CAD build for the part. Positions are in the model's coordinates, mm. Face numbers are marked on the shaded views. A direction names the side the tool comes from. Give positions to 0.01 mm unless a question says otherwise; leave off trailing zeros. Write each loop counter-clockwise with the first axis right and the second up, starting at its lowest first coordinate (ties: lowest second). Pieces come first, ordered by that corner, then holes. Notation, with made-up numbers: (28.5, 42.5) -> (56.5, 42.5) arc R24 ccw to (56.5, 65.5) -> close; hole circle Ø6 at (16, -36). An arc over 180 degrees is marked (long way). Answer in a Markdown table with one row per item. Add a question column.
Autodesk Inventor part; units mm, degrees
ref_plane "YZ Plane" through (0, 0, 0) normal (1, 0, 0) x (0, 1, 0)
ref_plane "XZ Plane" through (0, 0, 0) normal (0, 1, 0) x (-1, 0, 0)
ref_plane "XY Plane" through (0, 0, 0) normal (0, 0, 1) x (1, 0, 0)
sketch "Sketch1" plane through (0, 0, 0) normal (0, 1, 0) x (-1, 0, 0)
  line L0 (17.0295, 14.999) -> (-8.3705, 14.999)
  line L1 (-8.3705, 14.999) -> (-8.3705, -10.401)
  line L2 (-8.3705, -10.401) -> (17.0295, -10.401)
  line L3 (17.0295, -10.401) -> (17.0295, 14.999)
  line L4 (15.442, -8.8135) -> (-6.783, -8.8135)
  line L5 (-6.783, -8.8135) -> (-6.783, 13.4115)
  line L6 (-6.783, 13.4115) -> (15.442, 13.4115)
  line L7 (15.442, 13.4115) -> (15.442, -8.8135)
  point P0 (0, 0)
  dimension "d0" = 25.4
  dimension "d1" = 25.4
  dimension "d4" = 1.5875
  dimension "d5" = 1.5875
  dimension "d6" = 1.5875
  dimension "d7" = 1.5875
extrude "Extrusion2" add sketch "Sketch1" along normal blind 304.8
sketch "Sketch2" plane through (8.3705, 0, 14.999) normal (1, 0, 0) x (0, 0, -1)
  line L0 (0, 304.8) -> (25.4, 304.8)
  line L1 (25.4, 0) -> (25.4, 304.8)
  line L2 (0, 0) -> (0, 304.8)
  point P0 (14.999, 0)
  point P1 (19.05, 298.45)
  point P2 (19.05, 273.05)
  point P3 (6.35, 285.75)
  point P4 (6.35, 260.35)
  dimension "d10" = 6.35
  dimension "d11" = 6.35
  dimension "d12" = 6.35
  dimension "d13" = 25.4
  dimension "d14" = 6.35
  dimension "d15" = 25.4
  dimension "d16" = 6.35
  dimension "d17" = 19.05
hole "Hole1" at (8.3705, 298.45, -4.051) at (8.3705, 273.05, -4.051) at (8.3705, 285.75, 8.649) at (8.3705, 260.35, 8.649) direction (-1, 0, 0) diameter 4.7625 depth 25.4 tip angle 118
sketch "Sketch3" plane through (8.3705, 0, 14.999) normal (1, 0, 0) x (0, 0, -1)
  line L0 (25.4, 0) -> (25.4, 304.8)
  line L1 (0, 0) -> (25.4, 0)
  line L2 (0, 0) -> (0, 304.8)
  point P0 (14.999, 0)
  point P1 (6.35, 6.35)
  point P2 (19.05, 19.05)
  point P3 (6.35, 31.75)
  point P4 (19.05, 44.45)
  dimension "d25" = 6.35
  dimension "d26" = 6.35
  dimension "d27" = 19.05
  dimension "d28" = 25.4
  dimension "d29" = 6.35
  dimension "d30" = 6.35
  dimension "d31" = 6.35
  dimension "d32" = 25.4
hole "Hole2" at (8.3705, 6.35, 8.649) at (8.3705, 19.05, -4.051) at (8.3705, 31.75, 8.649) at (8.3705, 44.45, -4.051) direction (-1, 0, 0) diameter 4.7625 depth 25.4 tip angle 118
sketch "Sketch4" plane through (-17.0295, 0, 14.999) normal (0, 0, 1) x (1, 0, 0)
  line L0 (0, 0) -> (0, 304.8)
  line L1 (0, 0) -> (25.4, 0)
  line L2 (0, 304.8) -> (25.4, 304.8)
  point P0 (17.0295, 0)
  point P1 (12.7, 76.2)
  point P2 (12.7, 101.6)
  point P3 (12.7, 127)
  point P4 (12.7, 177.8)
  point P5 (12.7, 228.6)
  point P6 (12.7, 203.2)
  dimension "d40" = 12.7
  dimension "d41" = 12.7
  dimension "d42" = 12.7
  dimension "d43" = 25.4
  dimension "d44" = 25.4
  dimension "d45" = 76.2
  dimension "d46" = 12.7
  dimension "d47" = 12.7
  dimension "d48" = 12.7
  dimension "d49" = 25.4
  dimension "d50" = 25.4
  dimension "d51" = 76.2
hole "Hole3" at (-4.3295, 76.2, 14.999) at (-4.3295, 101.6, 14.999) at (-4.3295, 127, 14.999) at (-4.3295, 177.8, 14.999) at (-4.3295, 228.6, 14.999) at (-4.3295, 203.2, 14.999) direction (0, 0, -1) diameter 4.826 depth 25.4 tip angle 118.188
equation "\"d0\" = ElvBeamWidth"
equation "\"d1\" = ElvBeamWidth"
equation "\"d4\" = ElvWallWidth"
equation "\"d5\" = ElvWallWidth"
equation "\"d6\" = ElvWallWidth"
equation "\"d7\" = ElvWallWidth"
equation "\"d8\" = ElvCrossBeamLength"
equation "\"ElvMiddleBeamLength\" = 990.6"
equation "\"ElvWallWidth\" = 1.5875"
equation "\"ElvFrontBeamLength\" = 990.6"
equation "\"ElvEndEffectLength\" = 431.8"
equation "\"ElvCrossBeamLength\" = 304.8"
equation "\"ElvBeamWidth\" = 25.4"
equation "\"ElvFrontBeamLength_1\" = 1066.8"
equation "\"ElvFixedBeamLength\" = 990.6"
equation "\"ElvDelHeight\" = 101.6"
equation "\"ElvDelFrontTabLength\" = 6.35"
equation "\"ElvDelWidth\" = 18.542"
equation "\"ElvDelDepth\" = 6.35"
equation "\"ElvTopBeamLength\" = 457.2"
equation "\"ElvHoleFromBottom\" = 38.1"
equation "\"ElvHoleFromMid\" = 38.1"
equation "\"ElvHoleFromFixed\" = 50.8"
equation "\"ElvHoleFromFront\" = 25.4"
equation "\"ElvRivetPlateLength\" = 76.2"
equation "\"ElvDelMiddleTabLength\" = 6.35"
properties part number "ElvCrossBeam" material "Aluminum 6061"
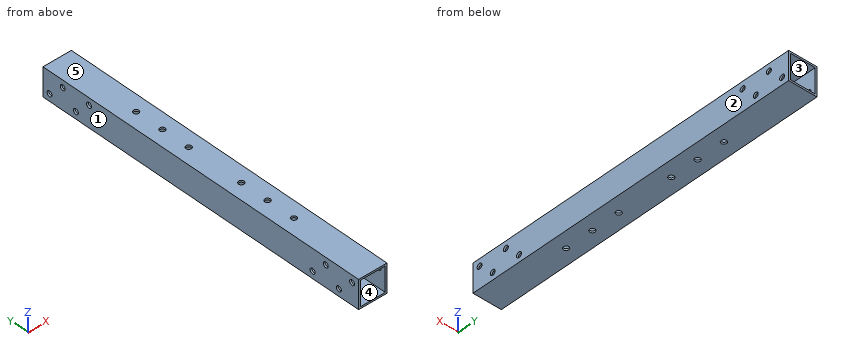
Item 1: Which spindle directions (+Z, -Z, +X, -X, +Y, -Y) get a long thin tool onto all of the face, cutting with end or side? Do the marked faces 4 and 5. Say none if no direction does.
Item 2: Slice it at A-A, the plane y = 152.5. List the corners of the cut face in (x, z), then the cut area to 3 significant figures.
Item 3: Drop a flat-ended pin along its axis: pin 1 Ø5.5 at (y, z) = (260.35, 8.649) entering from -X. Give the stop position or say it passes through.
Item 4: Probe L1, parallel to Z at x = -16.35, y = 260.35; L2, parallel to X at y = 46, z = 1.75; L3, parallel to X at y = 101.6, z = 14.75. List the from-to ranges inside material, lowest first. Write a range as from..to.
Item 5: Mould opens along X. For the marked faces 1, 2 and 3 say: released by +X, released by -X, zero draft, split by the parting line, or undercut.
Answer key:
| question | item | result |
|---|---|---|
| 1 | face 4 | +Y, -Y |
| 1 | face 5 | +Z, +X, -X, +Y, -Y |
| 2 | outline | (-17.03, -10.4) -> (8.37, -10.4) -> (8.37, 15) -> (-17.03, 15) -> close; hole (-15.44, -8.81) -> (6.78, -8.81) -> (6.78, 13.41) -> (-15.44, 13.41) -> close |
| 2 | area | 151 mm² |
| 3 | pin 1 | stops at x = -17.03 |
| 4 | L1 | z = -10.4..6.27, 11.03..15 |
| 4 | L2 | x = -17.03..-15.44, 6.78..8.37 |
| 4 | L3 | x = -17.03..-6.74, -1.92..8.37 |
| 5 | face 1 | released by -X |
| 5 | face 2 | released by +X |
| 5 | face 3 | undercut |
